The listing builds one solid part. Answer for the finished solid, in the listing's coordinates (mm). Give positions to 0.01 mm unless a question says otherwise; leave off trailing zeros.
Item 1: Consider line 1 along X through (y, z) = (65.5, 1.7); line 2 along Y through (x, z) = (15, 1.7); line 3 along X through (y, z) = (51, 2.1). Determine where each line is inside the solid, lowest interval first.
Item 2: Section A-A, the plane x = 5.08 is taken. Give the number of separate pieces and of enclosed holes in the cut face, and give its area (3 significant figures).
Item 3: Each of these flat-tipped pins is pushed along its axis until it touches: pin 1 Ø1 at (y, z) = (53.5, 0.5) entering from -X; pin 2 Ø3 at (x, y) = (43.18, 21.59) entering from -Z. Where does it stop, or does it pass through?
from build123d import *

# Parameters (mm, degrees)
F0_W     = 37.084
F0_H     = 86.36
F0_R     = 1.778
F0_R_2   = 6.35
F0_W_2   = 18.796
F1_DEPTH = 2.54


with BuildPart() as f1:
    # F0 (on Top) → F1 (new body)
    with BuildSketch(Plane.XY):
        with Locations((18.542, 43.18)):
            Rectangle(F0_W, F0_H)
        with Locations((5.08, 13.716)):
            Circle(F0_R, mode=Mode.SUBTRACT)
        with Locations((11.6332, 15.0368)):
            Circle(F0_R, mode=Mode.SUBTRACT)
        with Locations((11.6332, 20.2692)):
            Circle(F0_R, mode=Mode.SUBTRACT)
        with Locations((18.542, 17.399)):
            Circle(F0_R, mode=Mode.SUBTRACT)
        with Locations((25.4508, 15.0368)):
            Circle(F0_R, mode=Mode.SUBTRACT)
        with Locations((25.4508, 20.2692)):
            Circle(F0_R, mode=Mode.SUBTRACT)
        with Locations((5.08, 21.59)):
            Circle(F0_R, mode=Mode.SUBTRACT)
        with Locations((8.763, 27.178)):
            Circle(F0_R, mode=Mode.SUBTRACT)
        with Locations((5.08, 32.766)):
            Circle(F0_R, mode=Mode.SUBTRACT)
        with Locations((5.08, 40.64)):
            Circle(F0_R, mode=Mode.SUBTRACT)
        with Locations((11.6332, 34.0868)):
            Circle(F0_R, mode=Mode.SUBTRACT)
        with Locations((11.6332, 39.3192)):
            Circle(F0_R, mode=Mode.SUBTRACT)
        with Locations((18.542, 27.178)):
            Circle(F0_R_2, mode=Mode.SUBTRACT)
        with Locations((18.542, 36.957)):
            Circle(F0_R, mode=Mode.SUBTRACT)
        with Locations((25.4508, 34.0868)):
            Circle(F0_R, mode=Mode.SUBTRACT)
        with Locations((25.4508, 39.3192)):
            Circle(F0_R, mode=Mode.SUBTRACT)
        with Locations((32.004, 13.716)):
            Circle(F0_R, mode=Mode.SUBTRACT)
        with Locations((32.004, 21.59)):
            Circle(F0_R, mode=Mode.SUBTRACT)
        with Locations((28.321, 27.178)):
            Circle(F0_R, mode=Mode.SUBTRACT)
        with Locations((32.004, 32.766)):
            Circle(F0_R, mode=Mode.SUBTRACT)
        with Locations((32.004, 40.64)):
            Circle(F0_R, mode=Mode.SUBTRACT)
        with Locations((5.08, 51.816)):
            Circle(F0_R, mode=Mode.SUBTRACT)
        with Locations((11.6332, 53.1368)):
            Circle(F0_R, mode=Mode.SUBTRACT)
        with Locations((5.08, 59.69)):
            Circle(F0_R, mode=Mode.SUBTRACT)
        with Locations((11.6332, 58.3692)):
            Circle(F0_R, mode=Mode.SUBTRACT)
        with Locations((25.4508, 53.1368)):
            Circle(F0_R, mode=Mode.SUBTRACT)
        with Locations((18.542, 55.499)):
            Circle(F0_R, mode=Mode.SUBTRACT)
        with Locations((25.4508, 58.3692)):
            Circle(F0_R, mode=Mode.SUBTRACT)
        with Locations((5.08, 70.866)):
            Circle(F0_R, mode=Mode.SUBTRACT)
        with Locations((8.763, 65.278)):
            Circle(F0_R, mode=Mode.SUBTRACT)
        with Locations((11.6332, 72.1868)):
            Circle(F0_R, mode=Mode.SUBTRACT)
        with Locations((5.08, 78.74)):
            Circle(F0_R, mode=Mode.SUBTRACT)
        with Locations((11.6332, 77.4192)):
            Circle(F0_R, mode=Mode.SUBTRACT)
        with Locations((18.542, 65.278)):
            Circle(F0_R_2, mode=Mode.SUBTRACT)
        with Locations((18.542, 75.057)):
            Circle(F0_R, mode=Mode.SUBTRACT)
        with Locations((25.4508, 72.1868)):
            Circle(F0_R, mode=Mode.SUBTRACT)
        with Locations((25.4508, 77.4192)):
            Circle(F0_R, mode=Mode.SUBTRACT)
        with Locations((32.004, 51.816)):
            Circle(F0_R, mode=Mode.SUBTRACT)
        with Locations((32.004, 59.69)):
            Circle(F0_R, mode=Mode.SUBTRACT)
        with Locations((28.321, 65.278)):
            Circle(F0_R, mode=Mode.SUBTRACT)
        with Locations((32.004, 70.866)):
            Circle(F0_R, mode=Mode.SUBTRACT)
        with Locations((32.004, 78.74)):
            Circle(F0_R, mode=Mode.SUBTRACT)
        with Locations((46.482, 43.18)):
            Rectangle(F0_W_2, F0_H)
        with Locations((43.18, 13.716)):
            Circle(F0_R, mode=Mode.SUBTRACT)
        with Locations((49.7332, 15.0368)):
            Circle(F0_R, mode=Mode.SUBTRACT)
        with Locations((49.7332, 20.2692)):
            Circle(F0_R, mode=Mode.SUBTRACT)
        with Locations((43.18, 21.59)):
            Circle(F0_R, mode=Mode.SUBTRACT)
        with Locations((46.863, 27.178)):
            Circle(F0_R, mode=Mode.SUBTRACT)
        with Locations((43.18, 32.766)):
            Circle(F0_R, mode=Mode.SUBTRACT)
        with Locations((43.18, 40.64)):
            Circle(F0_R, mode=Mode.SUBTRACT)
        with Locations((49.7332, 34.0868)):
            Circle(F0_R, mode=Mode.SUBTRACT)
        with Locations((49.7332, 39.3192)):
            Circle(F0_R, mode=Mode.SUBTRACT)
        with Locations((43.18, 51.816)):
            Circle(F0_R, mode=Mode.SUBTRACT)
        with Locations((49.7332, 53.1368)):
            Circle(F0_R, mode=Mode.SUBTRACT)
        with Locations((43.18, 59.69)):
            Circle(F0_R, mode=Mode.SUBTRACT)
        with Locations((49.7332, 58.3692)):
            Circle(F0_R, mode=Mode.SUBTRACT)
        with Locations((46.863, 65.278)):
            Circle(F0_R, mode=Mode.SUBTRACT)
        with Locations((43.18, 70.866)):
            Circle(F0_R, mode=Mode.SUBTRACT)
        with Locations((49.7332, 72.1868)):
            Circle(F0_R, mode=Mode.SUBTRACT)
        with Locations((43.18, 78.74)):
            Circle(F0_R, mode=Mode.SUBTRACT)
        with Locations((49.7332, 77.4192)):
            Circle(F0_R, mode=Mode.SUBTRACT)
    extrude(amount=F1_DEPTH)


solid = f1.part
Worked answers:
1. line 1: x = 0 to 7, 10.53 to 12.2, 24.89 to 26.56, 30.09 to 45.1, 48.63 to 55.88
1. line 2: y = 0 to 21.91, 32.45 to 60.01, 70.55 to 86.36
1. line 3: x = 0 to 3.5, 6.66 to 30.42, 33.58 to 41.6, 44.76 to 55.88
2. separate pieces: 9
2. enclosed holes: 0
2. area: 147 mm2
3. pin 1: stops at x = 0
3. pin 2: passes through
